Model file for the job. Use its own axes, mm. A direction names the side the tool comes from. Coordinates: 2 decimals unless noted, no trailing zeros. Loops run counter-clockwise (first coordinate to the right, second up) from the corner with the lowest first, then second, coordinate; pieces in that order, holes last.
from build123d import *

# Parameters (mm, degrees)
F1_DEPTH  = 14
F2_R      = 1.65
F3_DEPTH  = 25
F4_R      = 6.99999
F5_R      = 1.125
F7_R      = 1.125
F9_W      = 14
F9_H      = 6.4348620027
F10_DEPTH = 29.7
F13_DEPTH = 1.1


# Not quite as in the source:
# - a fillet or chamfer is up to 0.001 mm smaller than in the source, because OpenCascade refuses the exact size


with BuildPart() as f1:
    # F0 (on Front) → F1 (new body)
    with BuildSketch(Plane.XZ):
        with BuildLine():
            ThreePointArc((-24.6100064665, 31.2714347113), (-31.6100064665, 38.2714347113), (-38.6100064665, 31.2714347113))
            Line((-38.6100064665, 31.2714347113), (-38.6100064665, 23.0214347113))
            Line((-38.6100064665, 23.0214347113), (-34.6100064665, 23.0214347113))
            Line((-34.6100064665, 23.0214347113), (-34.6100064665, 22.0214347113))
            Line((-34.6100064665, 22.0214347113), (-34.6100064665, 19.0214347113))
            Line((-34.6100064665, 19.0214347113), (-34.6100064665, 11.5214347113))
            Line((-34.6100064665, 11.5214347113), (-28.6100064665, 11.5214347113))
            Line((-28.6100064665, 11.5214347113), (-28.6100064665, 15.2714347113))
            Line((-28.6100064665, 15.2714347113), (-28.6100064665, 19.0214347113))
            Line((-28.6100064665, 19.0214347113), (-28.6100064665, 22.0214347113))
            Line((-28.6100064665, 22.0214347113), (-28.6100064665, 23.0214347113))
            Line((-28.6100064665, 23.0214347113), (-24.6100064665, 23.0214347113))
            Line((-24.6100064665, 23.0214347113), (-24.6100064665, 31.2714347113))
        make_face()
    extrude(amount=F1_DEPTH)

    # F2 (on face) → F3 (cut)
    with BuildSketch(Plane.YZ.offset(-28.6100064665)):
        with Locations((-7, 15.2714347113)):
            Circle(F2_R)
    extrude(amount=-F3_DEPTH, mode=Mode.SUBTRACT)

    # F4 (radius 7 in the source; OpenCascade refuses exactly that, so slightly less here)
    f4_edges = [f1.edges().sort_by_distance(p)[0] for p in [
        (-31.610006, -14, 11.521435),
        (-31.610006, 0, 11.521435),
    ]]
    fillet(f4_edges, radius=F4_R)

    # F5 (on face) → F6 (revolve)
    with BuildSketch(Plane.XZ.offset(14)):
        with Locations((-34.6100064665, 27.1464347113)):
            Circle(F5_R)
    revolve(axis=Axis((-31.6100064665, -14, 28.3964347113), (0, 0, -1)))

    # F7 (on face) → F8 (revolve)
    with BuildSketch(Plane(origin=(0, 0, 0), x_dir=(-1, 0, 0), z_dir=(0, 1, 0))):
        with Locations((28.6100064665, 27.1464347113)):
            Circle(F7_R)
    revolve(axis=Axis((-31.6100064665, 0, 28.3964347113), (0, 0, -1)))

    # F9 (on Top) → F10 (cut)
    with BuildSketch(Plane.XY):
        with Locations((-31.6100064665, -17.2174310014)):
            Rectangle(F9_W, F9_H)
    extrude(amount=F10_DEPTH, mode=Mode.SUBTRACT)

    # F12 (on offset) → F13 (cut, symmetric)
    with BuildSketch(Plane.YZ.offset(-31.5)):
        with BuildLine():
            ThreePointArc((-14, 31.6231168223), (-11.8, 27.3242797703), (-14, 23.0254427182))
            Line((-14, 23.0254427182), (-14, 20.4949313387))
            ThreePointArc((-14, 20.4949313387), (-9.6, 27.3242797703), (-14, 34.1536282018))
            Line((-14, 34.1536282018), (-14, 31.6231168223))
        make_face()
    extrude(amount=F13_DEPTH, both=True, mode=Mode.SUBTRACT)


solid = f1.part
Q1. Drill centre lines: line 1 (Z direction, x = -31.5, y = -7); line 2 (Y direction, x = -30.5, z = 27.25); line 3 (Y direction, x = -33.5, z = 19). Where is each one in solid material? Low to high.
Answers:
line 1: z = 11.52 to 13.62, 16.92 to 38.27
line 2: y = -14 to -11.8, -9.6 to 0, 1.52 to 3.97
line 3: y = -14 to 0
Q2. Which spindle directions (+Z, -Z, +X, -X, +Y, -Y) get a long thin tool onto all of the face, cutting with end or side? Do faces 1 (the cylindrical face through (-31.5, -9.6, 27.2)), 2 (the flat face through (-27, -7, 23.021)), 3 (the flat face through (-37, -7, 23.021)). Say none if no direction does.
Answers:
face 1: none
face 2: -Z, +X, +Y, -Y
face 3: -Z, -X, +Y, -Y
Q3. Mould opens along Z. For faces 4 (the cylindrical face through (-31.46, -6.9, 38.27)), 5 (the flat face through (-30.4, -11, 27)), 6 (the flat face through (-24.61, -7, 27)) say: +Z half, -Z half, draft (parallel to the pull), parting line (faces both ways), or undercut.
Answers:
face 4: +Z half
face 5: undercut
face 6: draft
Q4. Slice it at B-B (y = -6.25). List the corners of the cut face in (x, z), and give its area (3 significant figures).
Answers:
outline: (-38.61, 23.02) - (-34.61, 23.02) - (-34.61, 16.74) - (-28.61, 16.74) - (-28.61, 23.02) - (-24.61, 23.02) - (-24.61, 31.27) arc R7 ccw to (-38.61, 31.27) - close; (-34.61, 11.56) - (-28.61, 11.56) - (-28.61, 13.8) - (-34.61, 13.8) - close
area: 244 mm2
Q5. Slice it at D-D (y = -0.75). List the corners of the cut face in (x, z).
Answers:
outline: (-38.61, 23.02) - (-34.61, 23.02) - (-34.61, 15.37) - (-28.61, 15.37) - (-28.61, 23.02) - (-24.61, 23.02) - (-24.61, 31.27) arc R7 ccw to (-38.61, 31.27) - close
Q6. Slice it at C-C (y = -12.5). List the corners of the cut face in (x, z).
Answers:
outline: (-38.61, 23.02) - (-34.61, 23.02) - (-34.61, 14.19) - (-28.61, 14.19) - (-28.61, 23.02) - (-24.61, 23.02) - (-24.61, 31.27) arc R7 ccw to (-38.61, 31.27) - close; hole (-32.6, 21.4) - (-30.4, 21.4) - (-30.4, 24.69) - (-32.6, 24.69) - close; hole (-32.6, 29.96) - (-30.4, 29.96) - (-30.4, 33.25) - (-32.6, 33.25) - close
Q7. Flat gauge pins, fed straight in: P1, Ø4.5, axis at x = -26, y = -8, coming from the -Z side; P2, Ø3.5, axis at y = -6, z = 20, coming from the +X side; P3, Ø5.5, axis at y = -7, z = 15.27, coming from the -X side. Where does each tip first touch, or does it go through?
Answers:
P1: stops at z = 23.02
P2: stops at x = -28.61
P3: stops at x = -34.61
Q8. Slice it at A-A (z = 15.75). List the corners of the cut face in (x, y).
Answers:
outline: (-34.61, -13.43) - (-28.61, -13.43) - (-28.61, -8.58) - (-34.61, -8.58) - close; (-34.61, -5.42) - (-28.61, -5.42) - (-28.61, -0.57) - (-34.61, -0.57) - close
